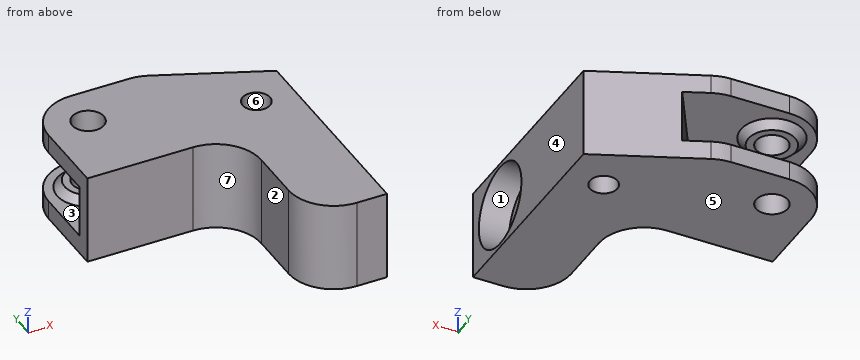
```python
from build123d import *

# Parameters (mm, degrees)
SKETCH1_R               = 1.822216084
SKETCH1_R_2             = 2.1
BOSS_EXTRUDE1_DEPTH     = 12
FILLET1_R               = 6
CUT_EXTRUDE1_DEPTH      = 3.5
CUT_EXTRUDE1_DEPTH_BACK = 3.5
SKETCH5_R               = 5.5
CUT_EXTRUDE2_DEPTH      = 4


with BuildPart() as part:
    # Sketch1 → Boss-Extrude1 (new body)
    with BuildSketch(Plane.XY):
        Polygon((15, 16), (30, 9.5), (30, -19), (20, -19), (20, 0), (0, 0), (0, 16), align=None)
        with Locations((25, 5)):
            Circle(SKETCH1_R, mode=Mode.SUBTRACT)
        with Locations((5.5, 10.5)):
            Circle(SKETCH1_R_2, mode=Mode.SUBTRACT)
    extrude(amount=BOSS_EXTRUDE1_DEPTH)

    # Fillet1
    fillet1_edges = [part.edges().sort_by_distance(p)[0] for p in [
        (0, 16, 6),
        (15, 16, 6),
        (20, -19, 6),
        (20, 0, 6),
    ]]
    fillet(fillet1_edges, radius=FILLET1_R)

    # Sketch2 → Cut-Extrude1 (cut, two sides: drawn at the far end of the back side and taken through both)
    with BuildSketch(Plane(origin=(0, 0, 6), x_dir=(-1, 0, 0), z_dir=(0, 0, -1)).offset(-CUT_EXTRUDE1_DEPTH_BACK)):
        Polygon((-22, 18.66922052), (-12, 2), (0, 2), (0, 22), align=None)
    extrude(amount=CUT_EXTRUDE1_DEPTH + CUT_EXTRUDE1_DEPTH_BACK, mode=Mode.SUBTRACT)

    # Sketch4 → Revolve1 (revolve)
    with BuildSketch(Plane(origin=(5.5, 0, 0), x_dir=(0, 0, -1), z_dir=(1, 0, 0)), mode=Mode.PRIVATE) as revolve1_sk:
        Polygon((-9.5, 12.6), (-8.5, 12.6), (-8.5, 13.6), (-9.5, 14.6), align=None)
    revolve1 = revolve(revolve1_sk.sketch.rotate(Axis((5.5, 10.5, 12), (0, 0, -1)), 90), axis=Axis((5.5, 10.5, 12), (0, 0, -1)))

    # Mirror1: Revolve1 across plane
    add(revolve1.mirror(Plane(origin=(0, 0, 6), x_dir=(1, 0, 0), z_dir=(0, 0, -1))))

    # Sketch5 → Cut-Extrude2 (cut)
    with BuildSketch(Plane(origin=(30, 0, 0), x_dir=(0, 0, -1), z_dir=(1, 0, 0))):
        with Locations((-6, -12)):
            Circle(SKETCH5_R)
    extrude(amount=-CUT_EXTRUDE2_DEPTH, mode=Mode.SUBTRACT)


solid = part.part
```
Design review of the part built by this model. Coordinates are the model's own, in mm. Face numbers are marked on the shaded views. A direction names the side the tool comes from. Round coordinates to 2 decimals unless told otherwise and drop trailing zeros. Order: outer loops, then holes, each group sorted by start corner. A loop starts at its lowest first (then second) coordinate and runs counter-clockwise, first axis right, second up. Notation, with made-up numbers: M -39.5,-32 L 5.5,-32 A22 ccw 5.5,-25 Z; hole C 11,83 d4. An arc over 180 degrees is marked long. Put each result on its own line as item: value.
Q1. Consider section D-D (y = 10.5). State the section outline as (x, z) points.
Reported:
outline: M 0.02,0 L 3.4,0 L 3.4,3.5 L 2.4,3.5 L 1.4,2.5 L 0.02,2.5 Z; M 0.02,9.5 L 1.4,9.5 L 2.4,8.5 L 3.4,8.5 L 3.4,12 L 0.02,12 Z; M 7.6,0 L 27.69,0 L 27.69,12 L 7.6,12 L 7.6,8.5 L 8.6,8.5 L 9.6,9.5 L 17.1,9.5 L 17.1,2.5 L 9.6,2.5 L 8.6,3.5 L 7.6,3.5 Z
Q2. Consider section C-C (y = -12). State the section outline as (x, z) points.
Reported:
outline: M 20,0 L 30,0 L 30,0.5 L 26,0.5 L 26,11.5 L 30,11.5 L 30,12 L 20,12 Z
Q3. Draft analysis for pull direction Y (two halves, no side actions). For the marked faces 5, 6 and 7, state which applies: released by +Y, released by -Y, zero draft, split by the parting line, or undercut.
Reported:
face 5: zero draft
face 6: undercut
face 7: released by -Y
Q4. Consider section A-A (z = 6). State the section outline as (x, y) points.
Reported:
outline: M 0,0 L 14,0 A6 cw 20,-6 L 20,-13 A6 ccw 26,-19 L 30,-19 L 30,-17.5 L 26,-17.5 L 26,-6.5 L 30,-6.5 L 30,9.5 L 19.28,14.14 L 12,2 L 0,2 Z; hole C 25,5 d3.64
Q5. To check wall thickness, follow line 1 (Z direction, x = 12.5, y = 8); line 2 (Y direction, x = 6, z = 9); line 3 (Y direction, x = 10, z = 11.5). State the ranges of each line that lie inside material, in increasing order.
Reported:
line 1: 0 to 2.5, 9.5 to 12
line 2: 0 to 2, 6.93 to 8.46, 12.54 to 14.07
line 3: 0 to 16
Q6. Machinability: for the marked faces 1, 2, 3 and 4, which of the approach directions +Z, -Z, +X, -X, +Y, -Y give a long, thin tool a straight path to every point of the face, cutting with its end or side? Answer none if there is none.
Reported:
face 1: +X
face 2: +Z, -Z, -X, -Y
face 3: none
face 4: +Z, -Z, +X, +Y, -Y
Q7. Insertion check: pin 1 Ø1.9 at (x, y) = (5.5, 10.5) entering from +Z; pin 2 Ø3.5 at (y, z) = (-10, 7.5) entering from -X; pin 3 Ø3.5 at (y, z) = (-10.5, 8.5) entering from +X; pin 4 Ø3.5 at (x, z) = (5, 5.5) entering from +Y. Each pin has a flat end and moves straight along its axis. Give the tip position at first contact, or say it passes through.
Reported:
pin 1: through
pin 2: x = 20
pin 3: x = 26
pin 4: y = 2
Q8. Consider section B-B (x = 5.5). State the section outline as (y, z) points, and give its area (3 significant figures).
Reported:
outline: M 0,0 L 8.4,0 L 8.4,3.5 L 7.4,3.5 L 6.4,2.5 L 2,2.5 L 2,9.5 L 6.4,9.5 L 7.4,8.5 L 8.4,8.5 L 8.4,12 L 0,12 Z; M 12.6,0 L 15.98,0 L 15.98,2.5 L 14.6,2.5 L 13.6,3.5 L 12.6,3.5 Z; M 12.6,8.5 L 13.6,8.5 L 14.6,9.5 L 15.98,9.5 L 15.98,12 L 12.6,12 Z
area: 78.9 mm²
